Work out the finished part from the listing and answer in its coordinate system (mm). Coordinates: 2 decimals unless noted, no trailing zeros. Order: outer loops, then holes, each group sorted by start corner. A loop starts at its lowest first (then second) coordinate and runs counter-clockwise, first axis right, second up. Notation, with made-up numbers: M 88,0.5 L 112,0.5 A17 cw 112,19.5 Z; hole C 21.5,75.5 d6. An arc over 180 degrees is marked long. Use a Markdown table: item, result.
from build123d import *

# Parameters (mm, degrees)
F0_R     = 1.75
F1_DEPTH = 5


with BuildPart() as f1:
    # F0 (on Top) → F1 (new body)
    with BuildSketch(Plane.XY):
        with BuildLine():
            Line((95, 0), (5, 0))
            ThreePointArc((5, 0), (1.4644660941, -1.4644660941), (0, -5))
            Line((0, -5), (0, -25))
            ThreePointArc((0, -25), (1.4644660941, -28.5355339059), (5, -30))
            Line((5, -30), (95, -30))
            ThreePointArc((95, -30), (98.5355339059, -28.5355339059), (100, -25))
            Line((100, -25), (100, -5))
            ThreePointArc((100, -5), (98.5355339059, -1.4644660941), (95, 0))
        make_face()
        Polygon((19.6251784864, -8.6899095669), (19.6251784864, -25), (17.7296525464, -25), (17.7296525464, -17.3250832937), (9.137315564, -17.3250832937), (9.137315564, -25), (7.241789624, -25), (7.241789624, -8.6899095669), (9.137315564, -8.6899095669), (9.137315564, -15.6294621609), (17.7296525464, -15.6294621609), (17.7296525464, -8.6899095669), align=None, mode=Mode.SUBTRACT)
        with BuildLine():
            Line((32.7118039029, -25), (31.3374583532, -25))
            Line((31.3374583532, -25), (30.969776297, -23.2579723941))
            Line((30.969776297, -23.2579723941), (30.8805330795, -23.2579723941))
            add(Edge.make_bspline(
                [(30.8805330795, -23.2579723941), (29.9666825321, -24.4074250357), (29.0581865778, -24.8161589719)],
                knots=[0, 0, 0, 1, 1, 1], degree=2))
            add(Edge.make_bspline(
                [(29.0581865778, -24.8161589719), (28.1496906235, -25.2248929081), (26.7860542599, -25.2248929081)],
                knots=[0, 0, 0, 1, 1, 1], degree=2))
            add(Edge.make_bspline(
                [(26.7860542599, -25.2248929081), (24.9690623513, -25.2248929081), (23.9374107568, -24.2860542599)],
                knots=[0, 0, 0, 1, 1, 1], degree=2))
            add(Edge.make_bspline(
                [(23.9374107568, -24.2860542599), (22.9057591623, -23.3472156116), (22.9057591623, -21.6194669205)],
                knots=[0, 0, 0, 1, 1, 1], degree=2))
            add(Edge.make_bspline(
                [(22.9057591623, -21.6194669205), (22.9057591623, -17.917658258), (28.8279390766, -17.7391718229)],
                knots=[0, 0, 0, 1, 1, 1], degree=2))
            Line((28.8279390766, -17.7391718229), (30.9019514517, -17.6713469776))
            Line((30.9019514517, -17.6713469776), (30.9019514517, -16.9109947644))
            add(Edge.make_bspline(
                [(30.9019514517, -16.9109947644), (30.9019514517, -15.472394098), (30.2843883865, -14.7870061875)],
                knots=[0, 0, 0, 1, 1, 1], degree=2))
            add(Edge.make_bspline(
                [(30.2843883865, -14.7870061875), (29.6668253213, -14.101618277), (28.3031889576, -14.101618277)],
                knots=[0, 0, 0, 1, 1, 1], degree=2))
            add(Edge.make_bspline(
                [(28.3031889576, -14.101618277), (26.7753450738, -14.101618277), (24.8476915754, -15.0368871966)],
                knots=[0, 0, 0, 1, 1, 1], degree=2))
            Line((24.8476915754, -15.0368871966), (24.2765349833, -13.6197049024))
            add(Edge.make_bspline(
                [(24.2765349833, -13.6197049024), (25.1796763446, -13.1306520704), (26.2559495478, -12.8522132318)],
                knots=[0, 0, 0, 1, 1, 1], degree=2))
            add(Edge.make_bspline(
                [(26.2559495478, -12.8522132318), (27.3322227511, -12.5737743931), (28.4174202761, -12.5737743931)],
                knots=[0, 0, 0, 1, 1, 1], degree=2))
            add(Edge.make_bspline(
                [(28.4174202761, -12.5737743931), (30.6020942408, -12.5737743931), (31.6569490719, -13.5429557354)],
                knots=[0, 0, 0, 1, 1, 1], degree=2))
            add(Edge.make_bspline(
                [(31.6569490719, -13.5429557354), (32.7118039029, -14.5121370776), (32.7118039029, -16.653974298)],
                knots=[0, 0, 0, 1, 1, 1], degree=2))
            Line((32.7118039029, -16.653974298), (32.7118039029, -25))
        make_face(mode=Mode.SUBTRACT)
        with BuildLine():
            Line((46.744407425, -25), (44.8917182294, -25))
            Line((44.8917182294, -25), (44.8917182294, -17.0894811994))
            add(Edge.make_bspline(
                [(44.8917182294, -17.0894811994), (44.8917182294, -15.5973346026), (44.2116849119, -14.8601856259)],
                knots=[0, 0, 0, 1, 1, 1], degree=2))
            add(Edge.make_bspline(
                [(44.2116849119, -14.8601856259), (43.5316515945, -14.1230366492), (42.0787720133, -14.1230366492)],
                knots=[0, 0, 0, 1, 1, 1], degree=2))
            add(Edge.make_bspline(
                [(42.0787720133, -14.1230366492), (40.1618277011, -14.1230366492), (39.2693955259, -15.1600428367)],
                knots=[0, 0, 0, 1, 1, 1], degree=2))
            add(Edge.make_bspline(
                [(39.2693955259, -15.1600428367), (38.3769633508, -16.1970490243), (38.3769633508, -18.585197525)],
                knots=[0, 0, 0, 1, 1, 1], degree=2))
            Line((38.3769633508, -18.585197525), (38.3769633508, -25))
            Line((38.3769633508, -25), (36.5242741552, -25))
            Line((36.5242741552, -25), (36.5242741552, -12.7736792004))
            Line((36.5242741552, -12.7736792004), (38.0306996668, -12.7736792004))
            Line((38.0306996668, -12.7736792004), (38.3305568777, -14.447881961))
            Line((38.3305568777, -14.447881961), (38.4198000952, -14.447881961))
            add(Edge.make_bspline(
                [(38.4198000952, -14.447881961), (38.9909566873, -13.5447405997), (40.0172536887, -13.046763446)],
                knots=[0, 0, 0, 1, 1, 1], degree=2))
            add(Edge.make_bspline(
                [(40.0172536887, -13.046763446), (41.0435506901, -12.5487862922), (42.3036649215, -12.5487862922)],
                knots=[0, 0, 0, 1, 1, 1], degree=2))
            add(Edge.make_bspline(
                [(42.3036649215, -12.5487862922), (44.5133269871, -12.5487862922), (45.6288672061, -13.6143503094)],
                knots=[0, 0, 0, 1, 1, 1], degree=2))
            add(Edge.make_bspline(
                [(45.6288672061, -13.6143503094), (46.744407425, -14.6799143265), (46.744407425, -17.0252260828)],
                knots=[0, 0, 0, 1, 1, 1], degree=2))
            Line((46.744407425, -17.0252260828), (46.744407425, -25))
        make_face(mode=Mode.SUBTRACT)
        with BuildLine():
            Line((69.1444550214, -12.7736792004), (71.0185625892, -12.7736792004))
            Line((71.0185625892, -12.7736792004), (71.0185625892, -20.7056163732))
            add(Edge.make_bspline(
                [(71.0185625892, -20.7056163732), (71.0185625892, -22.2013326987), (71.6985959067, -22.936696811)],
                knots=[0, 0, 0, 1, 1, 1], degree=2))
            add(Edge.make_bspline(
                [(71.6985959067, -22.936696811), (72.3786292242, -23.6720609234), (73.8279390766, -23.6720609234)],
                knots=[0, 0, 0, 1, 1, 1], degree=2))
            add(Edge.make_bspline(
                [(73.8279390766, -23.6720609234), (75.7484531176, -23.6720609234), (76.6337458353, -22.6243455497)],
                knots=[0, 0, 0, 1, 1, 1], degree=2))
            add(Edge.make_bspline(
                [(76.6337458353, -22.6243455497), (77.5190385531, -21.5766301761), (77.5190385531, -19.1991908615)],
                knots=[0, 0, 0, 1, 1, 1], degree=2))
            Line((77.5190385531, -19.1991908615), (77.5190385531, -12.7736792004))
            Line((77.5190385531, -12.7736792004), (79.3717277487, -12.7736792004))
            Line((79.3717277487, -12.7736792004), (79.3717277487, -25))
            Line((79.3717277487, -25), (77.8438838648, -25))
            Line((77.8438838648, -25), (77.5761542123, -23.3614945264))
            Line((77.5761542123, -23.3614945264), (77.4762018087, -23.3614945264))
            add(Edge.make_bspline(
                [(77.4762018087, -23.3614945264), (76.9086149453, -24.2646358877), (75.898381723, -24.7447643979)],
                knots=[0, 0, 0, 1, 1, 1], degree=2))
            add(Edge.make_bspline(
                [(75.898381723, -24.7447643979), (74.8881485007, -25.2248929081), (73.5923369824, -25.2248929081)],
                knots=[0, 0, 0, 1, 1, 1], degree=2))
            add(Edge.make_bspline(
                [(73.5923369824, -25.2248929081), (71.3612565445, -25.2248929081), (70.252855783, -24.1646834841)],
                knots=[0, 0, 0, 1, 1, 1], degree=2))
            add(Edge.make_bspline(
                [(70.252855783, -24.1646834841), (69.1444550214, -23.10447406), (69.1444550214, -20.7734412185)],
                knots=[0, 0, 0, 1, 1, 1], degree=2))
            Line((69.1444550214, -20.7734412185), (69.1444550214, -12.7736792004))
        make_face(mode=Mode.SUBTRACT)
        Polygon((56.59328891, -8.6899095669), (60.9126606378, -16.8467396478), (65.2605901951, -8.6899095669), (67.313184198, -8.6899095669), (61.8693479296, -18.6744407425), (61.8693479296, -25), (59.9524036173, -25), (59.9524036173, -18.76368396), (54.519276535, -8.6899095669), align=None, mode=Mode.SUBTRACT)
        with BuildLine():
            Line((93.5185625892, -25), (91.6658733936, -25))
            Line((91.6658733936, -25), (91.6658733936, -17.0894811994))
            add(Edge.make_bspline(
                [(91.6658733936, -17.0894811994), (91.6658733936, -15.5973346026), (90.9858400762, -14.8601856259)],
                knots=[0, 0, 0, 1, 1, 1], degree=2))
            add(Edge.make_bspline(
                [(90.9858400762, -14.8601856259), (90.3058067587, -14.1230366492), (88.8529271775, -14.1230366492)],
                knots=[0, 0, 0, 1, 1, 1], degree=2))
            add(Edge.make_bspline(
                [(88.8529271775, -14.1230366492), (86.9359828653, -14.1230366492), (86.0435506901, -15.1600428367)],
                knots=[0, 0, 0, 1, 1, 1], degree=2))
            add(Edge.make_bspline(
                [(86.0435506901, -15.1600428367), (85.151118515, -16.1970490243), (85.151118515, -18.585197525)],
                knots=[0, 0, 0, 1, 1, 1], degree=2))
            Line((85.151118515, -18.585197525), (85.151118515, -25))
            Line((85.151118515, -25), (83.2984293194, -25))
            Line((83.2984293194, -25), (83.2984293194, -12.7736792004))
            Line((83.2984293194, -12.7736792004), (84.804854831, -12.7736792004))
            Line((84.804854831, -12.7736792004), (85.1047120419, -14.447881961))
            Line((85.1047120419, -14.447881961), (85.1939552594, -14.447881961))
            add(Edge.make_bspline(
                [(85.1939552594, -14.447881961), (85.7651118515, -13.5447405997), (86.7914088529, -13.046763446)],
                knots=[0, 0, 0, 1, 1, 1], degree=2))
            add(Edge.make_bspline(
                [(86.7914088529, -13.046763446), (87.8177058544, -12.5487862922), (89.0778200857, -12.5487862922)],
                knots=[0, 0, 0, 1, 1, 1], degree=2))
            add(Edge.make_bspline(
                [(89.0778200857, -12.5487862922), (91.2874821514, -12.5487862922), (92.4030223703, -13.6143503094)],
                knots=[0, 0, 0, 1, 1, 1], degree=2))
            add(Edge.make_bspline(
                [(92.4030223703, -13.6143503094), (93.5185625892, -14.6799143265), (93.5185625892, -17.0252260828)],
                knots=[0, 0, 0, 1, 1, 1], degree=2))
            Line((93.5185625892, -17.0252260828), (93.5185625892, -25))
        make_face(mode=Mode.SUBTRACT)
        with Locations((5, -5)):
            Circle(F0_R, mode=Mode.SUBTRACT)
    extrude(amount=F1_DEPTH)


solid = f1.part
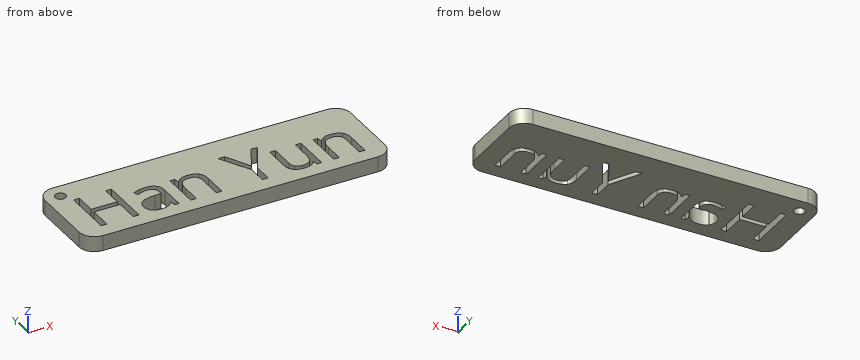
1. Section A-A on x = 14.5 is taken. Determine the outline of the cut face in (y, z).
Answers below:
| item | result |
|---|---|
| outline | M -30,0 L -17.33,0 L -17.33,5 L -30,5 Z; M -15.63,0 L 0,0 L 0,5 L -15.63,5 Z |
2. Section B-B on z = 3.2 is taken. Give the number of separate pieces and of enclosed holes in the cut face, then the cut area to 3 significant figures.
Answers below:
| item | result |
|---|---|
| separate pieces | 1 |
| enclosed holes | 7 |
| area | 2,600 mm² |
3. Find the intervals of material crossed by probe 1 along Y at (x, z) = (5, 3); probe 2 along Y at (x, z) = (74, 3.05); probe 3 along X at (y, z) = (-10, 4.25), in increasing order.
Answers below:
| item | result |
|---|---|
| probe 1 | -30 to -6.75, -3.25 to 0 |
| probe 2 | -30 to -25.21, -23.67 to 0 |
| probe 3 | 0 to 7.24, 9.14 to 17.73, 19.63 to 55.23, 57.29 to 64.56, 66.6 to 100 |
4. Section C-C on x = 59 is taken. Determine the outline of the cut face in (y, z), then the cut area to 3 significant figures.
Answers below:
| item | result |
|---|---|
| outline | M -30,0 L -17,0 L -17,5 L -30,5 Z; M -13.23,0 L 0,0 L 0,5 L -13.23,5 Z |
| area | 131 mm² |
5. A flat-ended cylindrical pin translates along its axis: P1, Ø3, axis at x = 5, y = -5, coming from the +Z side. Find the tip coordinate at first contact, or state that the pin passes through.
Answers below:
| item | result |
|---|---|
| P1 | through |
